Verification items for the finished model (mm, model axes). Face numbers are marked on the shaded views. Coordinates: 2 decimals unless noted, no trailing zeros. Loops run counter-clockwise (first coordinate to the right, second up) from the corner with the lowest first, then second, coordinate; pieces in that order, holes last. Notation, with made-up numbers: (67.5, 47) -> (95.5, 47) arc R36 cw to (95.5, 81) -> close; hole circle Ø9 at (58.25, 29). An arc over 180 degrees is marked (long way). Answer as a JSON object with one key per item and string values. Group by question number.
Q1. Release check for a two-part mould opening along X. For the marked faces 1, 2 and 3 record: released by +X, released by -X, zero draft, split by the parting line, or undercut.
Q2. Cross-section at C-C on x = 15. Record the boundary of the cut face in (y, z) (3 decimals), and give its area (3 significant figures).
Q3. Cross-section at A-A on x = 0. Record the boundary of the cut face in (y, z).
Q4. Gauge pin test, flat ends, axial feed: pin 1 Ø6.5 at (x, y) = (-15, 50) entering from -Z; pin 2 Ø5 at (x, z) = (-32, 3) entering from +Y; pin 3 Ø4 at (x, z) = (-32.5, 6.5) entering from -Y. Record the tip position at first contact, or that the pin passes through.
Q5. Cross-section at B-B on y = -21.5. Record the boundary of the cut face in (x, z).
Q6. Cross-section at D-D on x = -23. Record the boundary of the cut face in (y, z), and give its area (3 significant figures).
Q7. Scan lines: L1, parallel to X at y = 27.5, z = 5.25; L2, parallel to Y at x = 15, z = 2.25; L3, parallel to X at y = 8, z = 4. Record each from-to range of solid material in increasing order.
```python
from build123d import *

# Parameters (mm, degrees)
BOSS_EXTRUDE1_DEPTH            = 10.1
SKETCH3_W                      = 14.844682471
SKETCH3_H                      = 3
CUT_EXTRUDE1_DEPTH             = 73.814902321
M5_CLEARANCE_HOLE1_D           = 5.5
M5_CLEARANCE_HOLE1_CSINK_D     = 5.55
M5_CLEARANCE_HOLE1_CSINK_ANGLE = 90
FILLET1_R                      = 10
CUT_EXTRUDE2_DEPTH             = 87.915246219


with BuildPart() as part:
    # Sketch2 → Boss-Extrude1 (new body)
    with BuildSketch(Plane.XY):
        with BuildLine():
            Line((-40, 60), (-40, 0))
            ThreePointArc((-40, 0), (0, 40), (40, 0))
            Line((40, 0), (40, 60))
            Line((40, 60), (-40, 60))
        make_face()
        with BuildLine():
            ThreePointArc((40, 0), (0, 40), (-40, 0))
            Line((-40, 0), (-25.2, 0))
            ThreePointArc((-25.2, 0), (0, 25.2), (25.2, 0))
            Line((25.2, 0), (40, 0))
        make_face()
        with BuildLine():
            Line((-25.2, 0), (-40, 0))
            ThreePointArc((-40, 0), (0, -40), (40, 0))
            Line((40, 0), (25.2, 0))
            ThreePointArc((25.2, 0), (0, -25.2), (-25.2, 0))
        make_face()
    extrude(amount=BOSS_EXTRUDE1_DEPTH)

    # Sketch3 → Cut-Extrude1 (cut, through all)
    with BuildSketch(Plane.XY.offset(10.1)):
        with Locations((-32.577658765, 0)):
            Rectangle(SKETCH3_W, SKETCH3_H)
    extrude(amount=-CUT_EXTRUDE1_DEPTH, mode=Mode.SUBTRACT)

    # Sketch10 → CBORE for M5 SHCS3 (revolve, cut)
    with BuildSketch(Plane(origin=(-32.563591317, 60, 5.05), x_dir=(0, 0, 1), z_dir=(1, 0, 0))):
        Polygon((0, 0), (0, 100), (2.75, 100), (2.75, 10), (5, 10), (5, 0.025), (5.025, 0), align=None)
    revolve(axis=Axis((-32.563591317, 66.35, 5.05), (0, -1, 0)), mode=Mode.SUBTRACT)

    # M5 Clearance Hole1 (through all)
    with Locations(Plane.XY.offset(10.1)):
        with Locations((-15, 50), (15, 50)):
            CounterSinkHole(M5_CLEARANCE_HOLE1_D / 2, M5_CLEARANCE_HOLE1_CSINK_D / 2, counter_sink_angle=M5_CLEARANCE_HOLE1_CSINK_ANGLE)

    # Fillet1
    # the kernel refuses this fillet: 10 mm, written as the material it takes off along each edge
    with BuildSketch(Plane(origin=(-40, 60, -25), x_dir=(0, -1, 0), z_dir=(0, 0, 1))) as fillet1_piece_1:
        with BuildLine():
            CenterArc((FILLET1_R, FILLET1_R), FILLET1_R, 180, 90)
            Line((0, FILLET1_R), (0, 0))
            Line((0, 0), (FILLET1_R, 0))
        make_face()
    extrude(amount=60.1, mode=Mode.SUBTRACT)
    with BuildSketch(Plane(origin=(40, 60, -25), x_dir=(0, -1, 0), z_dir=(0, 0, 1))) as fillet1_piece_2:
        with BuildLine():
            CenterArc((FILLET1_R, -FILLET1_R), FILLET1_R, 90, 90)
            Line((0, -FILLET1_R), (0, 0))
            Line((0, 0), (FILLET1_R, 0))
        make_face()
    extrude(amount=60.1, mode=Mode.SUBTRACT)

    # Sketch18 → Cut-Extrude2 (cut, through all)
    with BuildSketch(Plane(origin=(0, -16.5, 0), x_dir=(1, 0, 0), z_dir=(0, 1, 0))):
        Polygon((-27.82931911, -5.05), (-30.196455214, -0.95), (-34.930727421, -0.95), (-37.297863525, -5.05), (-34.930727421, -9.15), (-30.196455214, -9.15), align=None)
    extrude(amount=-CUT_EXTRUDE2_DEPTH, mode=Mode.SUBTRACT)


solid = part.part
```
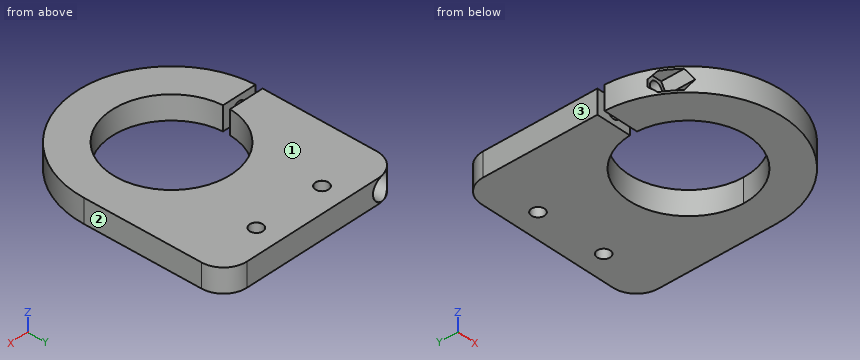
Computed values:
{
 "1": {"face 1": "zero draft", "face 2": "released by +X", "face 3": "released by -X"},
 "2": {"outline": "(-37.081, 0) -> (-20.249, 0) -> (-20.249, 10.1) -> (-37.081, 10.1) -> close; (20.249, 0) -> (47.25, 0) -> (47.25, 10.075) -> (47.225, 10.1) -> (20.249, 10.1) -> close; (52.75, 0) -> (60, 0) -> (60, 10.1) -> (52.775, 10.1) -> (52.75, 10.075) -> close", "area": "516 mm²"},
 "3": {"outline": "(-40, 0) -> (-25.2, 0) -> (-25.2, 10.1) -> (-40, 10.1) -> close; (25.2, 0) -> (60, 0) -> (60, 10.1) -> (25.2, 10.1) -> close"},
 "4": {"pin 1": "stops at z = 0", "pin 2": "stops at y = 50", "pin 3": "stops at y = -16.5"},
 "5": {"outline": "(-33.73, 0) -> (-13.14, 0) -> (-13.14, 10.1) -> (-33.73, 10.1) -> (-33.73, 9.15) -> (-30.2, 9.15) -> (-27.83, 5.05) -> (-30.2, 0.95) -> (-33.73, 0.95) -> close; (13.14, 0) -> (33.73, 0) -> (33.73, 10.1) -> (13.14, 10.1) -> close"},
 "6": {"outline": "(-32.73, 0) -> (-10.3, 0) -> (-10.3, 10.1) -> (-32.73, 10.1) -> close; (10.3, 0) -> (60, 0) -> (60, 10.1) -> (10.3, 10.1) -> close", "area": "729 mm²"},
 "7": {"L1": "x = -40 to -35.31, -29.82 to 40", "L2": "y = -37.08 to -20.25, 20.25 to 47.25, 52.75 to 60", "L3": "x = -40 to -35.11, -30.02 to -23.9, 23.9 to 40"}
}
